Check sheet for the modelled part. Datum: model origin and axes. Units: mm. Face numbers are marked on the shaded views. Give positions to 0.01 mm unless a question says otherwise; leave off trailing zeros. Write each loop counter-clockwise with the first axis right and the second up, starting at its lowest first coordinate (ties: lowest second). Pieces come first, ordered by that corner, then holes. Notation, with made-up numbers: (53, 9) -> (71, 9) arc R20 ccw to (71, 25) -> close; hole circle Ø11 at (36.25, 53). An arc over 180 degrees is marked (long way). Answer as a JSON object with one key per item and string values.
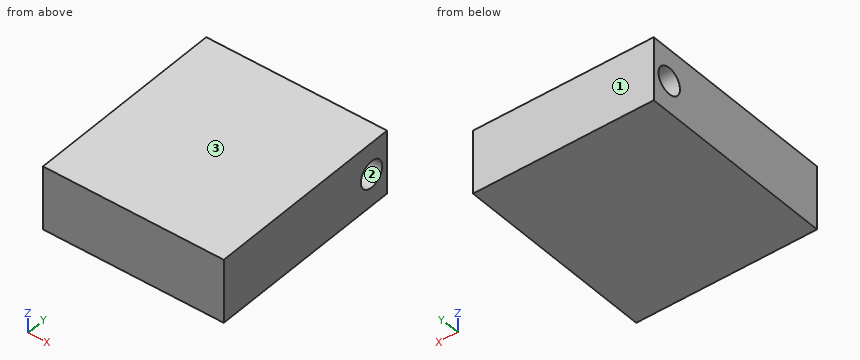
Autodesk Inventor part; units mm, degrees
ref_plane "YZ Plane" through (0, 0, 0) normal (1, 0, 0) x (0, 1, 0)
ref_plane "XZ Plane" through (0, 0, 0) normal (0, 1, 0) x (-1, 0, 0)
ref_plane "XY Plane" through (0, 0, 0) normal (0, 0, 1) x (1, 0, 0)
sketch "Esboço1" plane through (0, 0, 0) normal (0, 0, 1) x (1, 0, 0)
  circle A0 centre (0, 0) radius 68 construction
  line L0 (-42.5, 47.5) -> (42.5, 47.5)
  line L1 (42.5, -27.5) -> (42.5, -47.5)
  line L2 (42.5, -47.5) -> (-42.5, -47.5)
  line L3 (-42.5, -47.5) -> (-42.5, -27.5)
  line L4 (-42.5, 47.5) -> (42.5, -47.5) construction
  line L5 (42.5, 47.5) -> (-42.5, -47.5) construction
  line L6 (-42.5, -27.5) -> (-42.5, -12.5)
  line L7 (-42.5, -12.5) -> (-42.5, 47.5)
  line L8 (0, 106.3715) -> (0, -163.339) construction
  line L9 (42.5, -27.5) -> (42.5, -12.5)
  line L10 (42.5, -12.5) -> (42.5, 47.5)
  dimension "d0" = 136
  dimension "d1" = 85
  dimension "d2" = 95
  dimension "d13" = 20
  dimension "d14" = 60
  dimension "d15" = 42.5
extrude "Extrusão1" add sketch "Esboço1" along normal mid plane 30
sketch "Esboço2" plane through (42.5, -47.5, 15) normal (1, 0, 0) x (0, 0, -1)
  line L0 (30, 95) -> (0, 95) construction
  line L1 (15, 95) -> (15, 0) construction
  line L2 (30, 0) -> (0, 0) construction
  circle A0 centre (15, 86) radius 6.472 construction
  point P0 (15, 47.5)
  dimension "d5" = 9
hole "Furo1" at (42.5, 38.5, 0) direction (-1, 0, 0) diameter 12.5 end through all
properties part number "suporteGuiaCentralRetangular"
1. Mould release check, pull along Y, two halves, no side actions. Record for the marked faces 1, 2 and 3: released by +Y, released by -Y, zero draft, split by the parting line, or undercut.
Determined:
{"face 1": "released by +Y", "face 2": "undercut", "face 3": "zero draft"}
2. Sectioned sample at B-B, the plane y = 38.5. Enter the section's corners in (x, z).
Determined:
{"outline": "(-42.5, -15) -> (42.5, -15) -> (42.5, -6.25) -> (-42.5, -6.25) -> close; (-42.5, 6.25) -> (42.5, 6.25) -> (42.5, 15) -> (-42.5, 15) -> close"}
3. Scan lines: L1, parallel to Y at x = -12.5, z = 0; L2, parallel to Z at x = 20, y = 38.5; L3, parallel to Y at x = -8, z = -2.5. Record each from-to range of solid material in increasing order. Write a range as [from, to].
Determined:
{"L1": "[-47.5, 32.25], [44.75, 47.5]", "L2": "[-15, -6.25], [6.25, 15]", "L3": "[-47.5, 32.77], [44.23, 47.5]"}
4. Sectioned sample at A-A, the plane z = 0. Enter the section's corners in (x, y).
Determined:
{"outline": "(-42.5, -47.5) -> (42.5, -47.5) -> (42.5, 32.25) -> (-42.5, 32.25) -> close; (-42.5, 44.75) -> (42.5, 44.75) -> (42.5, 47.5) -> (-42.5, 47.5) -> close"}
5. Sectioned sample at C-C, the plane x = 10. Enter the section's corners in (y, z).
Determined:
{"outline": "(-47.5, -15) -> (47.5, -15) -> (47.5, 15) -> (-47.5, 15) -> close; hole circle Ø12.5 at (38.5, 0)"}
